from build123d import *

# Parameters (mm, degrees)
F0_R      = 60
F1_DEPTH  = 20
F2_R      = 29.25
F3_DEPTH  = 100
F4_R      = 25
F5_DEPTH  = 100
F6_W      = 5
F6_H      = 12
F7_DEPTH  = 100
F8_W      = 10
F8_H      = 7
F8_H_2    = 11
F9_DEPTH  = 12
F12_DEPTH = 2


with BuildPart() as f1:
    # F0 (on Top) → F1 (new body)
    with BuildSketch(Plane.XY):
        Circle(F0_R)
    extrude(amount=F1_DEPTH)

    # F2 (on face) → F3 (join)
    with BuildSketch(Plane(origin=(0, 0, 0), x_dir=(1, 0, 0), z_dir=(0, 0, -1))):
        Circle(F2_R)
    extrude(amount=F3_DEPTH)

    # F4 (on face) → F5 (cut)
    with BuildSketch(Plane(origin=(0, 0, -100), x_dir=(1, 0, 0), z_dir=(0, 0, -1))):
        Circle(F4_R)
    extrude(amount=-F5_DEPTH, mode=Mode.SUBTRACT)

    # F6 (on face) → F7 (join)
    with BuildSketch(Plane(origin=(0, 0, 0), x_dir=(1, 0, 0), z_dir=(0, 0, -1))):
        with Locations((-2.5, -34.831881)):
            Rectangle(F6_W, F6_H)
        with Locations((2.5, -34.831881)):
            Rectangle(F6_W, F6_H)
    extrude(amount=F7_DEPTH)

    # F8 (on face) → F9 (cut)
    with BuildSketch(Plane(origin=(0, 40.831881, 0), x_dir=(-1, 0, 0), z_dir=(0, 1, 0))):
        with Locations((0, -82.5)):
            Rectangle(F8_W, F8_H)
        with Locations((0, -62.5)):
            Rectangle(F8_W, F8_H)
        with Locations((0, -42.5)):
            Rectangle(F8_W, F8_H)
        with Locations((0, -22.5)):
            Rectangle(F8_W, F8_H)
        with Locations((0, -5.5)):
            Rectangle(F8_W, F8_H_2)
    extrude(amount=-F9_DEPTH, mode=Mode.SUBTRACT)

    # F11 (on offset) → F12 (cut)
    with BuildSketch(Plane.XZ.offset(-60)):
        Polygon((-8.660254, 17.5), (0, 2.5), (8.660254, 17.5), align=None)
    extrude(amount=F12_DEPTH, mode=Mode.SUBTRACT)


solid = f1.part
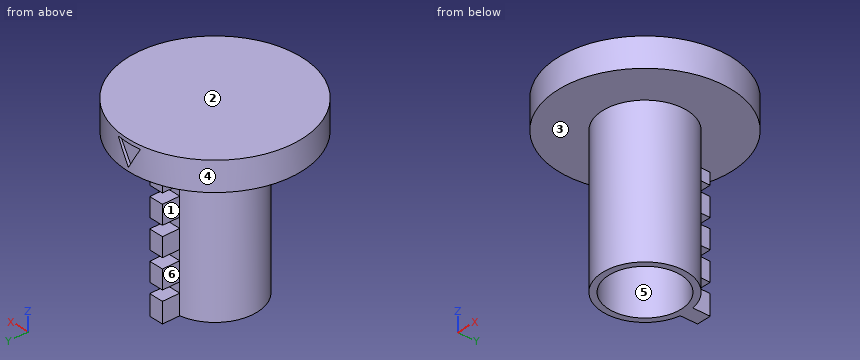
Verification items for the finished model (mm, model axes). Face numbers are marked on the shaded views. A direction names the side the tool comes from. Round coordinates to 2 decimals unless told otherwise and drop trailing zeros. Loops run counter-clockwise (first coordinate to the right, second up) from the corner with the lowest first, then second, coordinate; pieces in that order, holes last. Notation, with made-up numbers: M 57,80 L 95,80 A11 cw 95,92 Z; hole C -21.5,1.5 d5. An arc over 180 degrees is marked long. Write each question's results on one line, items separated by ' | '.
1) Gauge pin test, flat ends, axial feed: P1, Ø3, axis at x = -1, z = -4, coming from the +Y side; P2, Ø6.5, axis at y = 33, z = -15.5, coming from the +X side; P3, Ø6, axis at x = -1.5, z = -67, coming from the +Y side. Record the tip position at first contact, or that the pin passes through.
Checks:
P1: stops at y = 28.83 | P2: stops at x = 5 | P3: stops at y = 40.83
2) Scan lines: L1, parallel to Y at x = 0, z = -34.5; L2, parallel to Y at x = 0, z = -22; L3, parallel to Z at x = -49, y = 11. Record each from-to range of solid material in increasing order. Write a range as from..to.
Checks:
L1: y = -29.25..-25, 25..40.83 | L2: y = -29.25..-25, 25..28.83 | L3: z = 0..20
3) Section check C-C on x = 22.5. Record the boundary of the cut face in (y, z), then the cut area to 3 significant figures.
Checks:
outline: M -55.62,0 L -18.69,0 L -18.69,-100 L -10.9,-100 L -10.9,0 L 10.9,0 L 10.9,-100 L 18.69,-100 L 18.69,0 L 55.62,0 L 55.62,20 L -55.62,20 Z | area: 3,780 mm2
4) Access from +Z, -Z, +X, -X, +Y, -Y to the whole of each face (thin tool, end or side, straight path). Record for the marked faces 1 and 2.
Checks:
face 1: -Z, -X, +Y | face 2: +Z, +X, -X, +Y, -Y
5) Section check B-B on y = 0. Record the boundary of the cut face in (x, z), then the cut area to 3 significant figures.
Checks:
outline: M -60,0 L -29.25,0 L -29.25,-100 L -25,-100 L -25,0 L 25,0 L 25,-100 L 29.25,-100 L 29.25,0 L 60,0 L 60,20 L -60,20 Z | area: 3,250 mm2
6) Mould release check, pull along X, two halves, no side actions. Record for the marked faces 3, 4, 5 and 6: released by +X, released by -X, zero draft, split by the parting line, or undercut.
Checks:
face 3: zero draft | face 4: split by the parting line | face 5: undercut | face 6: released by -X
7) Section check D-D on z = -62. Record the boundary of the cut face in (x, y).
Checks:
outline: M -4.93,28.83 A29.25 ccw long 4.93,28.83 Z; hole C 0,0 d50
8) Section check A-A on z = -75.5. Record the boundary of the cut face in (x, y).
Checks:
outline: M -5,28.83 L -4.93,28.83 A29.25 ccw long 4.93,28.83 L 5,28.83 L 5,40.83 L -5,40.83 Z; hole C 0,0 d50
